Autodesk Inventor part; units mm, degrees
ref_plane "Work Plane1" through (0, 0, 45) normal (0, 0, 1) x (1, 0, 0)
ref_plane "YZ Plane" through (0, 0, 0) normal (1, 0, 0) x (0, 1, 0)
ref_plane "XZ Plane" through (0, 0, 0) normal (0, 1, 0) x (-1, 0, 0)
sketch "Sketch1" plane through (0, 0, 0) normal (0, 0, 1) x (1, 0, 0)
  line L0 (57.5, -28.5) -> (-57.5, -28.5)
  line L1 (-57.5, -28.5) -> (-57.5, 28.5)
  line L2 (-57.5, 28.5) -> (57.5, 28.5)
  line L3 (57.5, 28.5) -> (57.5, -28.5)
  line L4 (57.5, -28.5) -> (-57.5, 28.5) construction
  line L5 (-57.5, -28.5) -> (57.5, 28.5) construction
  line L6 (46.5, -16.5) -> (-46.5, -16.5) construction
  line L7 (-46.5, -16.5) -> (-46.5, 16.5) construction
  line L8 (-46.5, 16.5) -> (46.5, 16.5) construction
  line L9 (46.5, 16.5) -> (46.5, -16.5) construction
  line L10 (46.5, -16.5) -> (-46.5, 16.5) construction
  line L11 (-46.5, -16.5) -> (46.5, 16.5) construction
  line L12 (36, -11.5) -> (-36, -11.5) construction
  line L13 (-36, -11.5) -> (-36, 11.5) construction
  line L14 (-36, 11.5) -> (36, 11.5) construction
  line L15 (36, 11.5) -> (36, -11.5) construction
  line L16 (36, -11.5) -> (-36, 11.5) construction
  line L17 (-36, -11.5) -> (36, 11.5) construction
  circle A0 centre (-46.5, 16.5) radius 2.25
  circle A1 centre (-46.5, -16.5) radius 2.25
  circle A2 centre (46.5, -16.5) radius 2.25
  circle A3 centre (46.5, 16.5) radius 2.25
  point P0 (0, 0)
  dimension "d0" = 115
  dimension "d1" = 57
  dimension "d2" = 93
  dimension "d3" = 33
  dimension "d4" = 72
  dimension "d5" = 23
  dimension "d6" = 4.5
extrude "Extrusion1" add sketch "Sketch1" along normal blind 15
sketch "Sketch6" plane through (0, 0, 15) normal (0, 0, 1) x (1, 0, 0)
  line L0 (57.5, 28.5) -> (-57.5, 28.5)
  line L1 (28.5, -28.5) -> (-28.5, -28.5)
  line L2 (-28.5, -28.5) -> (-28.5, 28.5)
  line L3 (-28.5, 28.5) -> (28.5, 28.5)
  line L4 (28.5, 28.5) -> (28.5, -28.5)
  line L5 (28.5, -28.5) -> (-28.5, 28.5) construction
  line L6 (-28.5, -28.5) -> (28.5, 28.5) construction
  point P0 (0, 0)
  dimension "d27" = 57
ref_plane "Work Plane1" through (0, 0, 45) normal (0, 0, 1) x (1, 0, 0)
sketch "Sketch7" plane through (0, 0, 45) normal (0, 0, 1) x (1, 0, 0)
  line L0 (20.5, -20.5) -> (-20.5, -20.5)
  line L1 (-20.5, -20.5) -> (-20.5, 20.5)
  line L2 (-20.5, 20.5) -> (20.5, 20.5)
  line L3 (20.5, 20.5) -> (20.5, -20.5)
  line L4 (20.5, -20.5) -> (-20.5, 20.5) construction
  line L5 (-20.5, -20.5) -> (20.5, 20.5) construction
  point P0 (0, 0)
  dimension "d29" = 41
  dimension "d30" = 41
loft "Loft1" add profiles "Sketch6", "Sketch7"
fillet "Fillet2" radius 8 2 edges at (28.5, 0, 15) (-28.5, 0, 15)
sketch "Sketch8" plane through (0, 0, 0) normal (0, 1, 0) x (-1, 0, 0)
  line L0 (-34.6462, 15) -> (34.6462, 15)
  arc A0 (26.9163, 20.9387) -> (34.6462, 15) centre (34.6462, 23) ccw
  line L1 (26.9163, 20.9387) -> (20.5, 45)
  line L2 (20.5, 45) -> (-20.5, 45)
  line L3 (-26.9163, 20.9387) -> (-20.5, 45)
  arc A1 (-34.6462, 15) -> (-26.9163, 20.9387) centre (-34.6462, 23) ccw
  line L4 (57.5, 0) -> (-57.5, 0)
  line L5 (57.5, 0) -> (57.5, 15)
  line L6 (34.6462, 15) -> (57.5, 15)
  line L7 (-34.6462, 15) -> (34.6462, 15)
  line L8 (-57.5, 15) -> (-34.6462, 15)
  line L9 (-57.5, 0) -> (-57.5, 15)
  line L10 (57.5, 15) -> (24.1643, 31.2589)
  line L11 (26.9163, 20.9387) -> (20.5, 45)
  line L12 (24.1643, 31.2589) -> (24.1643, 15)
  line L13 (57.5, 0) -> (57.5, 15)
  line L14 (24.1643, 15) -> (57.5, 15)
  line L15 (-57.5, 15) -> (-24.1643, 31.2589)
  line L16 (-24.1643, 31.2589) -> (-24.1643, 15)
  line L17 (-34.6462, 15) -> (34.6462, 15)
  line L18 (-57.5, 15) -> (-34.6462, 15)
  line L19 (-24.1643, 15) -> (-57.5, 15)
  point P0 (0, 0)
  dimension "d36" = 26
  dimension "d37" = 26
extrude "Extrusion5" add sketch "Sketch8" along normal mid plane 15 contours A1 L3 L16 L0 | L8 L15 L3 A1 | L16 L3 L2 L1 L12 L0 | A0 L1 L10 L6
fillet "Fillet3" radius 8 4 edges at (-57.5, 28.5, 7.5) (-57.5, -28.5, 7.5) (57.5, -28.5, 7.5) (57.5, 28.5, 7.5)
sketch "Sketch9" plane through (0, 0, 0) normal (0, 1, 0) x (-1, 0, 0)
  line L0 (0, -9) -> (0, 54)
  line L1 (0, 0) -> (0, 45)
  line L2 (20.5, 45) -> (-20.5, 45)
  line L3 (0, 45) -> (-18.9, 45)
  line L4 (-18.9, 45) -> (-18.9, 15)
  line L5 (-18.9, 15) -> (-20.5, 15)
  line L6 (-20.5, 15) -> (-20.5, 0)
  line L7 (-20.5, 0) -> (0, 0)
  dimension "d41" = 37.8
  dimension "d42" = 41
  dimension "d43" = 15
revolve "Revolution2" cut sketch "Sketch9" angle 360 about axis through (0, 0, -10) along (0, 0, 1)
equation "\"d37\" = d36"
properties part number "sujetador guia ejercedor presion"
Could you check a few things on this model? Use its own coordinates, in mm. A direction names the side the tool comes from. Give positions to 0.01 mm unless a question says otherwise; leave off trailing zeros. Write each loop counter-clockwise with the first axis right and the second up, starting at its lowest first coordinate (ties: lowest second). Pieces come first, ordered by that corner, then holes. Notation, with made-up numbers: (-13, 29) -> (43, 29) arc R25 cw to (43, 47) -> close; hole circle Ø5 at (-16.5, -9.75). An arc over 180 degrees is marked (long way). Answer as CSV lines item,"result". Start each with the question number.
(1) Which directions (+Z, -Z, +X, -X, +Y, -Y) give clear straight access to the entire face, cutting with the end or side of a thin tool? Please do faces 1 (the face through (43, -18, 15)), 2 (the face through (-4.444, 20.013, 7.395)), 3 (the face through (-44, 18, 15)).
(2) If we section it at C-C, the plane y = -16.5: Give the number of separate pieces and of enclosed holes in the cut face, and give its area (3 significant figures).
(3) I'm going to push flat-ended pins straight in: pin 1 Ø2 at (x, z) = (-8.5, 23) entering from -Y; pin 2 Ø5 at (x, z) = (34.5, 21.5) entering from -Y; pin 3 Ø1 at (y, z) = (16, 20) entering from +X; pin 4 Ø3.5 at (x, y) = (46.5, 16.5) entering from -Z. Where does each tip first touch, or does it pass through?
(4) Please list where these lines run through material, in increasing order: line 1 (Y direction, x = -46.5, z = 5); line 2 (X direction, y = -16, z = 5); line 3 (Y direction, x = -48, z = 12).
(5) If we section it at B-B, the plane x = 46.5: Write out the boundary of the cut face in (y, z), and give its area (3 significant figures).
(6) If we section it at A-A, the plane y = 4: Write out the boundary of the cut face in (x, z).
(7) If we mould it in two halves opening along Y, with no side actions, what happens to faces 4 (the face through (18.027, -5.677, 29.79)), 5 (the face through (55.094, -26.219, 7.605)), 6 (the face through (-37, 7.5, 21)), 7 (the face through (18.4, 6.1, 45))? For each: +Y half, -Y half, draft (parallel to the pull), parting line (faces both ways), or undercut.
Answer list:
1,face 1,"+Z, +X, -Y"
1,face 2,"-Z"
1,face 3,"+Z, -X, +Y"
2,separate pieces,"4"
2,enclosed holes,"0"
2,area,"2,160 mm^2"
3,pin 1,"y = -26.63"
3,pin 2,"y = -7.5"
3,pin 3,"x = 27.45"
3,pin 4,"through"
4,line 1,"-28.5 to -18.75, -14.25 to 14.25, 18.75 to 28.5"
4,line 2,"-57.5 to -48.69, -44.31 to -12.82, 12.82 to 44.31, 48.69 to 57.5"
4,line 3,"-28.5 to -18.18, -14.82 to 14.82, 18.18 to 28.5"
5,outline,"(-28.5, 0) -> (-18.75, 0) -> (-18.75, 15) -> (-28.5, 15) -> close; (-14.25, 0) -> (14.25, 0) -> (14.25, 15) -> (7.5, 15) -> (7.5, 20.37) -> (-7.5, 20.37) -> (-7.5, 15) -> (-14.25, 15) -> close; (18.75, 0) -> (28.5, 0) -> (28.5, 15) -> (18.75, 15) -> close"
5,area,"800 mm^2"
6,outline,"(-57.5, 0) -> (-20.11, 0) -> (-20.11, 15) -> (-18.47, 15) -> (-18.47, 45) -> (-20.5, 45) -> (-24.16, 31.26) -> (-57.5, 15) -> close; (18.47, 15) -> (20.11, 15) -> (20.11, 0) -> (57.5, 0) -> (57.5, 15) -> (24.16, 31.26) -> (20.5, 45) -> (18.47, 45) -> close"
7,face 4,"undercut"
7,face 5,"-Y half"
7,face 6,"+Y half"
7,face 7,"draft"
